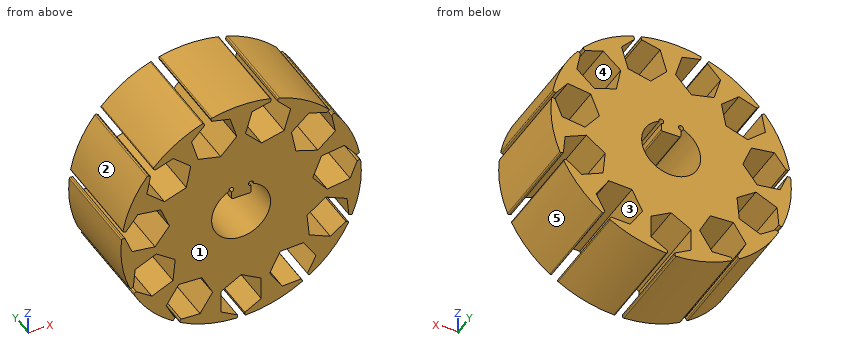
from build123d import *

# Parameters (mm, degrees)
SKETCH1_R                = 24.5
BOSS_EXTRUDE1_DEPTH      = 20
CUT_EXTRUDE1_DEPTH       = 41.006249512
FILLET1_R                = 0.25
CIRPATTERN1_COUNT        = 11
FILLET1_OF_CIRPATTERN1_R = 0.25
FILLET2_R                = 0.25


with BuildPart() as part:
    # Sketch1 → Boss-Extrude1 (new body)
    with BuildSketch(Plane(origin=(0, 0, 0), x_dir=(1, 0, 0), z_dir=(0, 1, 0))):
        with Locations(Location((0, 0, 0), (0, 0, 270))):
            Circle(SKETCH1_R)
        with BuildLine():
            Line((2, -5.167459748), (2, -3.51))
            Line((2, -3.51), (-2, -3.51))
            Line((-2, -3.51), (-2, -5.167459748))
            ThreePointArc((-2, -5.167459748), (-1.7197584, -6.081542645), (-2.464173015, -5.481601167))
            ThreePointArc((-2.464173015, -5.481601167), (0, 6.01), (2.464173015, -5.481601167))
            ThreePointArc((2.464173015, -5.481601167), (1.7197584, -6.081542645), (2, -5.167459748))
        make_face(mode=Mode.SUBTRACT)
    extrude(amount=BOSS_EXTRUDE1_DEPTH)

    # Sketch3 → Cut-Extrude1 (cut, through all)
    with BuildSketch(Plane(origin=(0, 20, 0), x_dir=(1, 0, 0), z_dir=(0, 1, 0))):
        Polygon((0.75, 23.801259505), (0.75, 24.5), (-0.75, 24.5), (-0.75, 23.801259505), (-4.1, 21.867136104), (-4.1, 17.132863896), (0, 14.765727793), (4.1, 17.132863896), (4.1, 21.867136104), align=None)
    cut_extrude1 = extrude(amount=-CUT_EXTRUDE1_DEPTH, mode=Mode.SUBTRACT)

    # Fillet1
    fillet1_edges = [part.edges().sort_by_distance(p)[0] for p in [
        (0.75, 10, -24.488517717),
        (-0.75, 10, -24.488517717),
    ]]
    fillet(fillet1_edges, radius=FILLET1_R)

    # CirPattern1: Cut-Extrude1 ×11 about axis
    cirpattern1_axis = Axis((0, 0, 0), (0, 1, 0))
    for i in range(1, CIRPATTERN1_COUNT):
        add(cut_extrude1.rotate(cirpattern1_axis, i * 360 / CIRPATTERN1_COUNT), mode=Mode.SUBTRACT)

    # Fillet1 of CirPattern1
    fillet1_of_cirpattern1_edges = [part.edges().sort_by_distance(p)[0] for p in [
        (-12.608552087, 10, -21.006532657),
        (-13.870432387, 10, -20.195571431),
        (-21.963977975, 10, -10.855121903),
        (-22.587100494, 10, -9.490673909),
        (-24.345996045, 10, 2.742713357),
        (-24.132523788, 10, 4.22744552),
        (-18.998332392, 10, 15.469756505),
        (-18.016041291, 10, 16.603380866),
        (-7.61883244, 10, 23.285261267),
        (-6.17959298, 10, 23.707860102),
        (6.17959298, 10, 23.707860102),
        (7.61883244, 10, 23.285261267),
        (18.016041291, 10, 16.603380866),
        (18.998332392, 10, 15.469756505),
        (24.132523788, 10, 4.22744552),
        (24.345996045, 10, 2.742713357),
        (22.587100494, 10, -9.490673909),
        (21.963977975, 10, -10.855121903),
        (13.870432387, 10, -20.195571431),
        (12.608552087, 10, -21.006532657),
    ]]
    fillet(fillet1_of_cirpattern1_edges, radius=FILLET1_OF_CIRPATTERN1_R)

    # Fillet2
    fillet2_edges = [part.edges().sort_by_distance(p)[0] for p in [
        (-2, 10, 3.51),
        (2, 10, 3.51),
    ]]
    fillet(fillet2_edges, radius=FILLET2_R)


solid = part.part
The listing builds one solid part. Answer for the finished solid, in the listing's coordinates (mm). Face numbers are marked on the shaded views. A direction names the side the tool comes from. Round coordinates to 2 decimals unless told otherwise and drop trailing zeros. Order: outer loops, then holes, each group sorted by start corner. A loop starts at its lowest first (then second) coordinate and runs counter-clockwise, first axis right, second up. Notation, with made-up numbers: (76, 84.5) - (90, 84.5) arc R21 cw to (90, 101.5) - close; hole circle Ø11 at (49.5, 77.25). An arc over 180 degrees is marked (long way). Write item = value, one per line. Start each with the question number.
1) Given pin 1 (4 mm diameter, centred on y = 5.5, z = -18.5, fed in from -X); pin 2 (3 mm diameter, centred on x = -18.5, y = 16, fed in from -Z); pin 3 (5 mm diameter, centred on y = 3, z = -9, fed in from -X), each flat-ended and moving along its own axis, determine where each tip first touches the part or whether it passes through.
2) For the marked faces 4 and 5, determine the directions among +Z, -Z, +X, -X, +Y, -Y from which every point of the face is accessible in a straight line to the end or side of a thin tool.
3) Section C-C, the plane z = 9 is taken. Write down the section's boundary in (x, y), plus the area to 3 significant figures.
4) Straight lines are drawn through the part: L1, parallel to X at y = 9.25, z = 14; L2, parallel to X at y = 12, z = -14; L3, parallel to X at y = 16.75, z = 2. For each, find the intervals that lie inside material, in ascending order.
5) Section A-A, the plane z = 21 is taken. Write down the section's boundary in (x, y), plus the area to 3 significant figures.
6) Section B-B, the plane z = 0 is taken. Write down the section's boundary in (x, y).
7) For a pull along Z with two mould halves and no side action, classify the marked faces 1, 2 and 3 as released by +Z, released by -Z, zero draft, split by the parting line, or undercut.
Results list:
q1.pin_1 = -18.11
q1.pin_2 = -17.64
q1.pin_3 = -23.62
q2.face_4 = +Y, -Y
q2.face_5 = -Z, +X, +Y, -Y
q3.outline = (-22.79, 0) - (-16.65, 0) - (-16.65, 20) - (-22.79, 20) - close; (-13.09, 0) - (13.09, 0) - (13.09, 20) - (-13.09, 20) - close; (16.65, 0) - (22.79, 0) - (22.79, 20) - (16.65, 20) - close
q3.area = 769 mm^2
q4.L1 = -20.11 to -18.68, -10.32 to 10.32, 18.68 to 20.11
q4.L2 = -20.11 to -13.87, -7.17 to 7.17, 13.87 to 20.11
q4.L3 = -24.42 to -23.41, -14.7 to -5.67, 5.67 to 14.7, 23.41 to 24.42
q5.outline = (-12.62, 0) - (-8.98, 0) - (-8.98, 20) - (-12.62, 20) - close; (-1.89, 0) - (1.89, 0) - (1.89, 20) - (-1.89, 20) - close; (8.98, 0) - (12.62, 0) - (12.62, 20) - (8.98, 20) - close
q5.area = 221 mm^2
q6.outline = (-24.5, 0) - (-22.61, 0) - (-22.61, 20) - (-24.5, 20) - close; (-16.27, 0) - (-6.01, 0) - (-6.01, 20) - (-16.27, 20) - close; (6.01, 0) - (16.27, 0) - (16.27, 20) - (6.01, 20) - close; (22.61, 0) - (24.5, 0) - (24.5, 20) - (22.61, 20) - close
q7.face_1 = zero draft
q7.face_2 = released by +Z
q7.face_3 = undercut
